The listing builds one solid part. Answer for the finished solid, in the listing's coordinates (mm). Face numbers are marked on the shaded views. A direction names the side the tool comes from. Coordinates: 2 decimals unless noted, no trailing zeros. Order: outer loops, then holes, each group sorted by start corner. A loop starts at its lowest first (then second) coordinate and runs counter-clockwise, first axis right, second up. Notation, with made-up numbers: (4.5, 81.25) -> (10.5, 81.25) arc R19 ccw to (10.5, 92.25) -> close; hole circle Ø2 at (-2, 10.25). An arc over 180 degrees is marked (long way). Answer in a Markdown table with one row per item. Add a question column.
```python
from build123d import *

# Parameters (mm, degrees)
SKETCH1_R           = 21
BOSS_EXTRUDE1_DEPTH = 45
SKETCH2_R           = 6.5
BOSS_EXTRUDE2_DEPTH = 15
SKETCH3_R           = 25
BOSS_EXTRUDE3_DEPTH = 9
CUT_EXTRUDE1_REACH  = 92.25
SKETCH5_R           = 12
CHAMFER1_SIZE       = 2.5
CHAMFER1_SIZE2      = 0.669872981


with BuildPart() as part:
    # Sketch1 → Boss-Extrude1 (new body)
    with BuildSketch(Plane(origin=(0, 0, 0), x_dir=(1, 0, 0), z_dir=(0, 1, 0))):
        with Locations(Location((0, 0, 0), (0, 0, 90))):
            Circle(SKETCH1_R)
    extrude(amount=BOSS_EXTRUDE1_DEPTH)

    # Sketch2 → Boss-Extrude2 (add)
    with BuildSketch(Plane(origin=(0, 45, 0), x_dir=(1, 0, 0), z_dir=(0, 1, 0))):
        with BuildLine():
            ThreePointArc((-57.496195447, -9.157943365), (-60, 0), (-57.496195447, 9.157943365))
            ThreePointArc((-57.496195447, 9.157943365), (0, 36), (57.496195447, 9.157943365))
            ThreePointArc((57.496195447, 9.157943365), (60, 0), (57.496195447, -9.157943365))
            ThreePointArc((57.496195447, -9.157943365), (0, -36), (-57.496195447, -9.157943365))
        make_face()
        with Locations(Location((-42, 0, 0), (0, 0, 270))):
            Circle(SKETCH2_R, mode=Mode.SUBTRACT)
        with Locations(Location((42, 0, 0), (0, 0, 90))):
            Circle(SKETCH2_R, mode=Mode.SUBTRACT)
    extrude(amount=BOSS_EXTRUDE2_DEPTH)

    # Sketch3 → Boss-Extrude3 (add)
    with BuildSketch(Plane(origin=(0, 60, 0), x_dir=(1, 0, 0), z_dir=(0, 1, 0))):
        with Locations(Location((0, 0, 0), (0, 0, 270))):
            Circle(SKETCH3_R)
    extrude(amount=BOSS_EXTRUDE3_DEPTH)

    # Sketch4 → Cut-Revolve1 (revolve, cut)
    with BuildSketch(Plane.XY):
        with BuildLine():
            Line((-12, 57), (0, 57))
            Line((0, 57), (0, 69))
            Line((0, 69), (-23, 69))
            ThreePointArc((-23, 69), (-19.845922252, 60.849571269), (-12, 57))
        make_face()
    revolve(axis=Axis((0, 69, 0), (0, -1, 0)), mode=Mode.SUBTRACT)

    # Sketch5 → Cut-Extrude1 (cut, up to next)
    with BuildSketch(Plane(origin=(0, 57, 0), x_dir=(1, 0, 0), z_dir=(0, 1, 0)), mode=Mode.PRIVATE) as cut_extrude1_sk1:
        with Locations(Location((0, 0, 0), (0, 0, 180))):
            Circle(SKETCH5_R)
    cut_extrude1_tool1 = extrude(cut_extrude1_sk1.sketch, amount=-CUT_EXTRUDE1_REACH, mode=Mode.PRIVATE) & part.part
    add(cut_extrude1_tool1.solids().sort_by_distance((0, 57, 0))[0], mode=Mode.SUBTRACT)

    # Chamfer1
    chamfer1_edges = [part.edges().sort_by_distance(p)[0] for p in [
        (12, 0, 0),
    ]]
    chamfer1_side = [part.faces().sort_by_distance(p)[0] for p in [
        (0, 0, 20.406030304),
    ]]
    chamfer(chamfer1_edges, length=CHAMFER1_SIZE, length2=CHAMFER1_SIZE2, reference=chamfer1_side[0])


solid = part.part
```
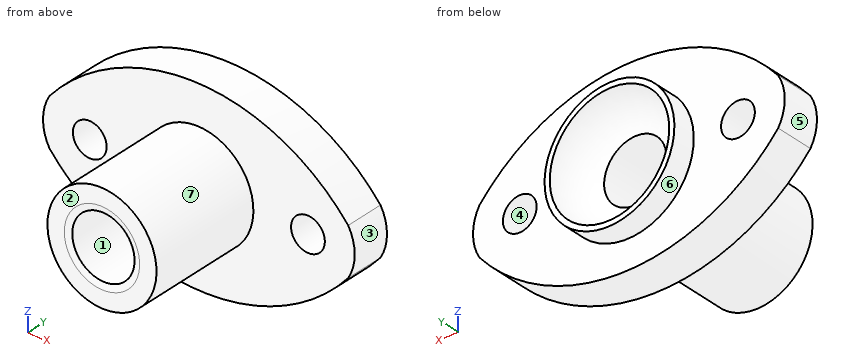
Q1. A cutting plane is placed at C-C (y = 11). Determine the outline of the cut face in (x, z).
Q2. For the marked faces 5, 6 and 7, determine the directions among +Z, -Z, +X, -X, +Y, -Y from which every point of the face is accessible in a straight line to the end or side of a thin tool.
Q3. Determine the mould class of the marked faces 1, 2, 3 and 4 for opening direction Z: +Z half, -Z half, draft (parallel to the pull), parting line (faces both ways), or undercut.
Q4. Given pin 1 (21.5 mm diameter, centred on x = 0, z = 0, fed in from +Y); pin 2 (2 mm diameter, centred on x = 28, z = -20, fed in from -Y); pin 3 (3 mm diameter, centred on x = 26.5, z = -2.5, fed in from +Y); pin 4 (21.5 mm diameter, centred on x = -28, z = -12, fed in from -Y), each flat-ended and moving along its own axis, determine where each tip first touches the part or whether it passes through.
Q5. A cutting plane is placed at A-A (x = -44.5). Determine the outline of the cut face in (y, z).
Q6. Straight lines are drawn through the part: line 1 (X direction, y = 44.5, z = 0); line 2 (Y direction, x = 37, z = -20.5); line 3 (X direction, y = 62, z = 5). For each, find the intervals that lie inside material, in ascending order.
Q7. A cutting plane is placed at D-D (x = 42). Determine the outline of the cut face in (y, z), then the cut area to 3 significant figures.
Q8. A cutting plane is placed at B-B (z = 0). State how many separate pieces and enclosed holes the cut face has, then the cut area to 3 significant figures.
Returned:
| question | item | result |
|---|---|---|
| 1 | outline | circle Ø42 at (0, 0); hole circle Ø24 at (0, 0) |
| 2 | face 5 | -X, +Y, -Y |
| 2 | face 6 | +Y |
| 2 | face 7 | -Y |
| 3 | face 1 | undercut |
| 3 | face 2 | draft |
| 3 | face 3 | parting line |
| 3 | face 4 | undercut |
| 4 | pin 1 | passes through |
| 4 | pin 2 | stops at y = 45 |
| 4 | pin 3 | stops at y = 60 |
| 4 | pin 4 | stops at y = 0 |
| 5 | outline | (45, -21.37) -> (60, -21.37) -> (60, -6) -> (45, -6) -> close; (45, 6) -> (60, 6) -> (60, 21.37) -> (45, 21.37) -> close |
| 6 | line 1 | x = -21 to -12, 12 to 21 |
| 6 | line 2 | y = 45 to 60 |
| 6 | line 3 | x = -24.49 to -20.17, 20.17 to 24.49 |
| 7 | outline | (45, -23.14) -> (60, -23.14) -> (60, -6.5) -> (45, -6.5) -> close; (45, 6.5) -> (60, 6.5) -> (60, 23.14) -> (45, 23.14) -> close |
| 7 | area | 499 mm² |
| 8 | separate pieces | 4 |
| 8 | enclosed holes | 0 |
| 8 | area | 1,890 mm² |
